The listing builds one solid part. Answer for the finished solid, in the listing's coordinates (mm). A direction names the side the tool comes from. Coordinates: 2 decimals unless noted, no trailing zeros. Order: outer loops, then holes, each group sorted by start corner. A loop starts at its lowest first (then second) coordinate and runs counter-clockwise, first axis right, second up. Notation, with made-up numbers: (63.5, 69) -> (75.5, 69) arc R11 ccw to (75.5, 84) -> close; hole circle Ø4 at (-6.5, -22.5). An arc over 180 degrees is marked (long way). Answer in a Markdown table with one row per item.
```python
from build123d import *

# Parameters (mm, degrees)
SKETCH3_W               = 101.6
SKETCH3_H               = 75
BOSS_EXTRUDE2_DEPTH     = 55
CUT_EXTRUDE2_DEPTH      = 122.465262524
CUT_EXTRUDE2_DEPTH_BACK = 122.465262524
SKETCH4_R               = 34.361552214
BOSS_EXTRUDE4_DEPTH     = 101.6
BOSS_EXTRUDE5_DEPTH     = 101.6
CUT_EXTRUDE3_DEPTH      = 125.423596536
CUT_EXTRUDE3_DEPTH_BACK = 125.423596536
SKETCH9_W               = 91.6
SKETCH9_H               = 49
SKETCH11_R              = 8.637348936
SKETCH11_R_2            = 6.137348936
BOSS_EXTRUDE6_DEPTH     = 2.5
FILLET2_R               = 1
BOSS_EXTRUDE7_START     = -2.5
BOSS_EXTRUDE7_DEPTH     = 2.5
FILLET3_R               = 1
CUT_EXTRUDE4_START      = -10
SKETCH13_R              = 2.5
CUT_EXTRUDE4_DEPTH      = 12.5
CUT_EXTRUDE5_START      = -7.5
SKETCH14_R              = 2.5
CUT_EXTRUDE5_DEPTH      = 10
LPATTERN2_COUNT         = 4
LPATTERN2_PITCH         = 20
LPATTERN3_COUNT         = 4
LPATTERN3_PITCH         = 20


with BuildPart() as part:
    # Sketch3 → Boss-Extrude2 (new body)
    with BuildSketch(Plane(origin=(0, 0, 0), x_dir=(1, 0, 0), z_dir=(0, 1, 0))):
        Rectangle(SKETCH3_W, SKETCH3_H)
    extrude(amount=BOSS_EXTRUDE2_DEPTH)

    # Sketch4 → Cut-Extrude2 (cut, two sides: drawn at the far end of the back side and taken through both)
    with BuildSketch(Plane(origin=(50.8, 0, 0), x_dir=(0, 0, -1), z_dir=(1, 0, 0)).offset(-CUT_EXTRUDE2_DEPTH_BACK)):
        with Locations((0, 55)):
            Circle(SKETCH4_R)
    extrude(amount=CUT_EXTRUDE2_DEPTH + CUT_EXTRUDE2_DEPTH_BACK, mode=Mode.SUBTRACT)

    # Sketch7 → Boss-Extrude4 (add)
    with BuildSketch(Plane.ZY.offset(50.8)):
        Polygon((-37.5, 55), (-63.5, 0), (-37.5, 0), align=None)
    extrude(amount=-BOSS_EXTRUDE4_DEPTH)

    # Sketch8 → Boss-Extrude5 (add)
    with BuildSketch(Plane.ZY.offset(50.8)):
        Polygon((37.5, 55), (61.876010058, 0), (37.5, 0), align=None)
    extrude(amount=-BOSS_EXTRUDE5_DEPTH)

    # Sketch9 → Cut-Extrude3 (cut, two sides: drawn at the far end of the back side and taken through both)
    with BuildSketch(Plane(origin=(0, 0, -37.5), x_dir=(-1, 0, 0), z_dir=(0, 0, -1)).offset(-CUT_EXTRUDE3_DEPTH_BACK)):
        with Locations((0, 27.5)):
            Rectangle(SKETCH9_W, SKETCH9_H)
    extrude(amount=CUT_EXTRUDE3_DEPTH + CUT_EXTRUDE3_DEPTH_BACK, mode=Mode.SUBTRACT)

    # Sketch11 → Boss-Extrude6 (add)
    with BuildSketch(Plane(origin=(0, 55, 0), x_dir=(1, 0, 0), z_dir=(0, 1, 0))):
        with Locations((0, 42.107585669)):
            Circle(SKETCH11_R)
        with Locations((0, 42.107585669)):
            Circle(SKETCH11_R_2, mode=Mode.SUBTRACT)
    extrude(amount=-BOSS_EXTRUDE6_DEPTH)

    # Fillet2
    # the kernel refuses this fillet: 1 mm, written as the material it takes off along each edge
    with BuildSketch(Plane(origin=(0, 52.5, -42.107585669), x_dir=(0.7661198217735417, 0, 0.6426977662056067), z_dir=(-0.6426977662056067, 0, 0.7661198217735417))) as fillet2_piece_1_section:
        with BuildLine():
            CenterArc((8.637348936 - FILLET2_R, FILLET2_R), FILLET2_R, 270, 90)
            Line((8.637348936, FILLET2_R), (8.637348936, 0))
            Line((8.637348936, 0), (8.637348936 - FILLET2_R, 0))
        make_face()
    fillet2_piece_1 = revolve(axis=Axis((0, 52.5, -42.107585669), (0, 1, 0)), revolution_arc=259.986561096, mode=Mode.PRIVATE)
    fillet2_piece_1 = split(fillet2_piece_1, bisect_by=Plane(origin=(0, 51.176344905, -39.307546045), z_dir=(0, 0.42737961689341614, -0.9040722665053037)), keep=Keep.TOP, mode=Mode.PRIVATE)
    add(fillet2_piece_1, mode=Mode.SUBTRACT)
    with BuildSketch(Plane(origin=(0, 55, -42.107585669), x_dir=(0.6577465140217427, 0, 0.753239353255156), z_dir=(-0.753239353255156, 0, 0.6577465140217427))) as fillet2_piece_2_section:
        with BuildLine():
            CenterArc((8.637348936 - FILLET2_R, -FILLET2_R), FILLET2_R, 0, 90)
            Line((8.637348936 - FILLET2_R, 0), (8.637348936, 0))
            Line((8.637348936, 0), (8.637348936, -FILLET2_R))
        make_face()
    fillet2_piece_2 = revolve(axis=Axis((0, 55, -42.107585669), (0, 1, 0)), revolution_arc=277.743530493, mode=Mode.PRIVATE)
    fillet2_piece_2 = split(fillet2_piece_2, bisect_by=Plane(origin=(0, 53.219711563, -38.341590898), z_dir=(0, 0.42737961689341614, -0.9040722665053037)), keep=Keep.TOP, mode=Mode.PRIVATE)
    add(fillet2_piece_2, mode=Mode.SUBTRACT)

    # Boss-Extrude7: read off the stored shape, not the designer's step
    # Boss-Extrude7 outline → Boss-Extrude7 (add)
    with BuildSketch(Plane(origin=(0, 55, 0), x_dir=(1, 0, 0), z_dir=(0, 1, 0)).offset(BOSS_EXTRUDE7_START)):
        with BuildLine():
            Line((-50.8, -34.361552214), (-50.8, -37.5))
            Line((-50.8, -37.5), (-7.182675213, -37.5))
            ThreePointArc((-7.182675213, -37.5), (0, -49.257807046), (7.182675213, -37.5))
            Line((7.182675213, -37.5), (50.8, -37.5))
            Line((50.8, -37.5), (50.8, -34.361552214))
            Line((50.8, -34.361552214), (4.313996334, -34.361552214))
            ThreePointArc((4.313996334, -34.361552214), (0, -33.11220702), (-4.313996334, -34.361552214))
            Line((-4.313996334, -34.361552214), (-50.8, -34.361552214))
        make_face()
        with BuildLine():
            ThreePointArc((4.180529051, -37.5), (0, -46.757807046), (-4.180529051, -37.5))
            Line((-4.180529051, -37.5), (4.180529051, -37.5))
        make_face(mode=Mode.SUBTRACT)
    extrude(amount=BOSS_EXTRUDE7_DEPTH)

    # Fillet3
    # the kernel refuses this fillet: 1 mm, written as the material it takes off along each edge
    with BuildSketch(Plane(origin=(0, 52.5, 41.185007033), x_dir=(-0.8048848647873229, 0, -0.5934310022540891), z_dir=(0.5934310022540891, 0, -0.8048848647873229))) as fillet3_piece_1_section:
        with BuildLine():
            CenterArc((8.072800013 - FILLET3_R, FILLET3_R), FILLET3_R, 270, 90)
            Line((8.072800013 - FILLET3_R, 0), (8.072800013, 0))
            Line((8.072800013, 0), (8.072800013, FILLET3_R))
        make_face()
    fillet3_piece_1 = revolve(axis=Axis((0, 52.5, 41.185007033), (0, 1, 0)), revolution_arc=252.801724897, mode=Mode.PRIVATE)
    fillet3_piece_1 = split(fillet3_piece_1, bisect_by=Plane(origin=(0, 51.545382329, 39.031087184), z_dir=(0, 0.4051883376708072, 0.9142332366609561)), keep=Keep.TOP, mode=Mode.PRIVATE)
    add(fillet3_piece_1, mode=Mode.SUBTRACT)
    with BuildSketch(Plane(origin=(0, 55, 41.185007033), x_dir=(-0.7077045492924725, 0, -0.7065085073166059), z_dir=(0.7065085073166059, 0, -0.7077045492924725))) as fillet3_piece_2_section:
        with BuildLine():
            CenterArc((8.072800013 - FILLET3_R, -FILLET3_R), FILLET3_R, 0, 90)
            Line((8.072800013, -FILLET3_R), (8.072800013, 0))
            Line((8.072800013, 0), (8.072800013 - FILLET3_R, 0))
        make_face()
    fillet3_piece_2 = revolve(axis=Axis((0, 55, 41.185007033), (0, 1, 0)), revolution_arc=269.903086539, mode=Mode.PRIVATE)
    fillet3_piece_2 = split(fillet3_piece_2, bisect_by=Plane(origin=(0, 53.634938356, 38.10499557), z_dir=(0, 0.4051883376708072, 0.9142332366609561)), keep=Keep.TOP, mode=Mode.PRIVATE)
    add(fillet3_piece_2, mode=Mode.SUBTRACT)

    # Sketch13 → Cut-Extrude4 (cut)
    with BuildSketch(Plane(origin=(0, 3, 0), x_dir=(1, 0, 0), z_dir=(0, 1, 0)).offset(CUT_EXTRUDE4_START)):
        with Locations(Location((-35.8, -50.546409509, 0), (0, 0, 90))):
            Circle(SKETCH13_R)
    cut_extrude4 = extrude(amount=CUT_EXTRUDE4_DEPTH, mode=Mode.SUBTRACT)

    # Sketch14 → Cut-Extrude5 (cut)
    with BuildSketch(Plane(origin=(0, 3, 0), x_dir=(1, 0, 0), z_dir=(0, 1, 0)).offset(CUT_EXTRUDE5_START)):
        with Locations(Location((-35.8, 52.081818182, 0), (0, 0, 90))):
            Circle(SKETCH14_R)
    cut_extrude5 = extrude(amount=CUT_EXTRUDE5_DEPTH, mode=Mode.SUBTRACT)

    # LPattern2: Cut-Extrude4 ×4
    with Locations(*[(i * LPATTERN2_PITCH, 0, 0) for i in range(1, LPATTERN2_COUNT)]):
        add(cut_extrude4, mode=Mode.SUBTRACT)

    # LPattern3: Cut-Extrude5 ×4
    with Locations(*[(i * LPATTERN3_PITCH, 0, 0) for i in range(1, LPATTERN3_COUNT)]):
        add(cut_extrude5, mode=Mode.SUBTRACT)


solid = part.part
```
(1) A flat-ended cylindrical pin translates along its axis: pin 1 (8 mm diameter, centred on x = -34.5, y = 6.5, fed in from -Z). Find the tip coordinate at first contact, or state that the pin passes through.
Check values:
| item | result |
|---|---|
| pin 1 | z = -62.32 |
(2) A cutting plane is placed at D-D, the plane y = 37. Determine the outline of the cut face in (x, z).
Check values:
| item | result |
|---|---|
| outline | (-50.8, -46.01) -> (-45.8, -46.01) -> (-45.8, -29.27) -> (-50.8, -29.27) -> close; (-50.8, 29.27) -> (-45.8, 29.27) -> (-45.8, 45.48) -> (-50.8, 45.48) -> close; (45.8, -46.01) -> (50.8, -46.01) -> (50.8, -29.27) -> (45.8, -29.27) -> close; (45.8, 29.27) -> (50.8, 29.27) -> (50.8, 45.48) -> (45.8, 45.48) -> close |
(3) A cutting plane is placed at A-A, the plane x = 10.5. Determine the outline of the cut face in (y, z), then the cut area to 3 significant figures.
Check values:
| item | result |
|---|---|
| outline | (0, -63.5) -> (3, -62.08) -> (3, 60.55) -> (0, 61.88) -> close; (52, -38.92) -> (55, -37.5) -> (55, -34.36) arc R34.36 cw to (52, -34.23) -> close; (52, 34.23) arc R34.36 cw to (55, 34.36) -> (55, 37.5) -> (52, 38.83) -> close |
| area | 395 mm² |
(4) Find the intervals of material crossed by line 1 along X through (y, z) = (9, -35.5); line 2 along Y through (x, z) = (-3, 6.5), in increasing order. Write a range as from..to.
Check values:
| item | result |
|---|---|
| line 1 | -50.8..-45.8, 45.8..50.8 |
| line 2 | 0..3 |
(5) Which of the six approach directions +Z, -Z, +X, -X, +Y, -Y give full straight-line access (tool end or side, diameter ignored) to faces 4 (the cylindrical face through (5.16, 1.48, -54.39)), 5 (the cylindrical face through (-34.84, 1.48, -54.39)), 6 (the flat face through (1, 52, 37))?
Check values:
| item | result |
|---|---|
| face 4 | -Y |
| face 5 | +Y, -Y |
| face 6 | +Z, -Z |
(6) A cutting plane is placed at B-B, the plane x = 24.2. Determine the outline of the cut face in (y, z), then the cut area to 3 significant figures.
Check values:
| item | result |
|---|---|
| outline | (0, -63.5) -> (3, -62.08) -> (3, -54.58) -> (0, -54.58) -> close; (0, -49.58) -> (3, -49.58) -> (3, 48.05) -> (0, 48.05) -> close; (0, 53.05) -> (3, 53.05) -> (3, 60.55) -> (0, 61.88) -> close; (52, -38.92) -> (55, -37.5) -> (55, -34.36) arc R34.36 cw to (52, -34.23) -> close; (52, 34.23) arc R34.36 cw to (55, 34.36) -> (55, 37.5) -> (52, 38.83) -> close |
| area | 365 mm² |
(7) A cutting plane is placed at C-C, the plane z = 0. Determine the outline of the cut face in (x, y), then the cut area to 3 significant figures.
Check values:
| item | result |
|---|---|
| outline | (-50.8, 0) -> (50.8, 0) -> (50.8, 20.64) -> (45.8, 20.64) -> (45.8, 3) -> (-45.8, 3) -> (-45.8, 20.64) -> (-50.8, 20.64) -> close |
| area | 481 mm² |
(8) For a pull along X with two mould halves and no side action, classify faces 1 (the flat face through (-50.8, 16, 0)), 2 (the flat face through (45.8, 16, 0)), 3 (the flat face through (0, 55, 36)) as released by +X, released by -X, zero draft, split by the parting line, or undercut.
Check values:
| item | result |
|---|---|
| face 1 | released by -X |
| face 2 | undercut |
| face 3 | zero draft |
